Read the model definition and answer for the solid it produces. Units are mm, in the model's axes. Face numbers are marked on the shaded views. A direction names the side the tool comes from. Coordinates: 2 decimals unless noted, no trailing zeros. Loops run counter-clockwise (first coordinate to the right, second up) from the corner with the lowest first, then second, coordinate; pieces in that order, holes last. Notation, with made-up numbers: (-31, 45) -> (-26, 45) arc R7 cw to (-26, 51) -> close; hole circle Ø7 at (-13.75, -13). An arc over 180 degrees is marked (long way). Answer in a Markdown table with one row per item.
```python
from build123d import *

# Parameters (mm, degrees)
ESBO_O1_R                = 17.5
RESSALTO_EXTRUS_O1_DEPTH = 5
ESBO_O2_R                = 10
RESSALTO_EXTRUS_O2_DEPTH = 10
ESBO_O3_R                = 4
CORTE_EXTRUS_O1_DEPTH    = 16
ESBO_O4_R                = 1.5
CORTE_EXTRUS_O2_DEPTH    = 10
ESBO_O5_R                = 1.5
CORTE_EXTRUS_O3_DEPTH    = 18.5
ESBO_O6_R                = 1.5
CORTE_EXTRUS_O4_DEPTH    = 18.5


with BuildPart() as part:
    # Esboço1 → Ressalto-extrusão1 (new body)
    with BuildSketch(Plane(origin=(0, 0, 0), x_dir=(1, 0, 0), z_dir=(0, 1, 0))):
        Circle(ESBO_O1_R)
    extrude(amount=RESSALTO_EXTRUS_O1_DEPTH)

    # Esboço2 → Ressalto-extrusão2 (add)
    with BuildSketch(Plane(origin=(0, 5, 0), x_dir=(1, 0, 0), z_dir=(0, 1, 0))):
        Circle(ESBO_O2_R)
    extrude(amount=RESSALTO_EXTRUS_O2_DEPTH)

    # Esboço3 → Corte-extrusão1 (cut, through all)
    with BuildSketch(Plane(origin=(0, 15, 0), x_dir=(1, 0, 0), z_dir=(0, 1, 0))):
        Circle(ESBO_O3_R)
    extrude(amount=-CORTE_EXTRUS_O1_DEPTH, mode=Mode.SUBTRACT)

    # Esboço4 → Corte-extrusão2 (cut)
    with BuildSketch(Plane(origin=(0, 5, 0), x_dir=(1, 0, 0), z_dir=(0, 1, 0))):
        with Locations((0, 13.75)):
            Circle(ESBO_O4_R)
        with Locations((0, -13.75)):
            Circle(ESBO_O4_R)
    extrude(amount=-CORTE_EXTRUS_O2_DEPTH, mode=Mode.SUBTRACT)

    # Esboço5 → Corte-extrusão3 (cut, through all)
    with BuildSketch(Plane.XY):
        with Locations((0, 10)):
            Circle(ESBO_O5_R)
    extrude(amount=-CORTE_EXTRUS_O3_DEPTH, mode=Mode.SUBTRACT)

    # Esboço6 → Corte-extrusão4 (cut, through all)
    with BuildSketch(Plane(origin=(0, 0, 0), x_dir=(0, 0, -1), z_dir=(1, 0, 0))):
        with Locations((0, 10)):
            Circle(ESBO_O6_R)
    extrude(amount=-CORTE_EXTRUS_O4_DEPTH, mode=Mode.SUBTRACT)


solid = part.part
```
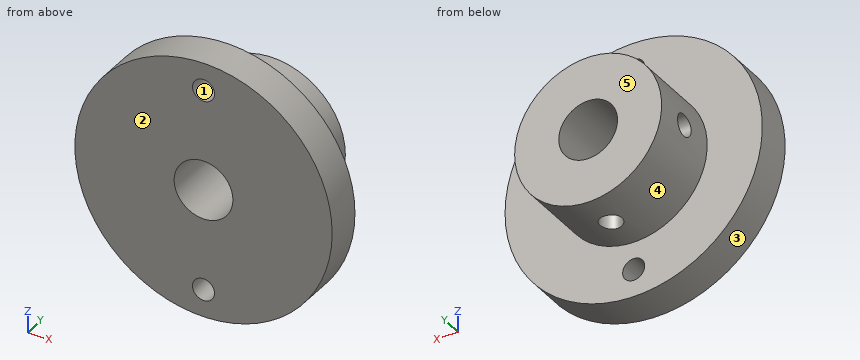
1. A tool of negligible diameter and unlimited length cuts with its end or side. For the marked faces 4 and 5, from which of +Z, -Z, +X, -X, +Y, -Y can it reach the whole face along a straight path? Write none if from no direction.
A:
| item | result |
|---|---|
| face 4 | +Y |
| face 5 | +Z, -Z, +X, -X, +Y |
2. A cutting plane is placed at B-B on x = 0. Give the vertices of the cut face in (y, z).
A:
| item | result |
|---|---|
| outline | (0, -17.5) -> (5, -17.5) -> (5, -15.25) -> (0, -15.25) -> close; (0, -12.25) -> (5, -12.25) -> (5, -10) -> (8.5, -10) -> (8.5, -4) -> (0, -4) -> close; (0, 4) -> (15, 4) -> (15, 10) -> (5, 10) -> (5, 12.25) -> (0, 12.25) -> close; (0, 15.25) -> (5, 15.25) -> (5, 17.5) -> (0, 17.5) -> close; (11.5, -10) -> (15, -10) -> (15, -4) -> (11.5, -4) -> close |
3. The mould has two halves that part along X. Classify the marked faces 1, 2 and 3: pulls with the +X half, pulls with the -X half, needs draft (parallel to the pull), parting line crosses it, or undercut.
A:
| item | result |
|---|---|
| face 1 | undercut |
| face 2 | needs draft |
| face 3 | parting line crosses it |
4. A cutting plane is placed at C-C on y = 10. Give the vertices of the cut face in (x, z).
A:
| item | result |
|---|---|
| outline | (-9.89, -1.5) arc R10 ccw to (-1.5, -9.89) -> (-1.5, -3.71) arc R4 cw to (-3.71, -1.5) -> close; (-9.89, 1.5) -> (-3.71, 1.5) arc R4 cw (long way) to (1.5, -3.71) -> (1.5, -9.89) arc R10 ccw (long way) to start |
5. Find the intervals of material crossed by probe 1 along Z at (x, y) = (0, 3.7); probe 2 along Y at (x, z) = (0, -8); probe 3 along Y at (x, z) = (-10, 13), in increasing order.
A:
| item | result |
|---|---|
| probe 1 | z = -17.5 to -15.25, -12.25 to -4, 4 to 12.25, 15.25 to 17.5 |
| probe 2 | y = 0 to 8.5, 11.5 to 15 |
| probe 3 | y = 0 to 5 |
6. A cutting plane is placed at D-D on z = 14.5. Give the vertices of the cut face in (x, y).
A:
| item | result |
|---|---|
| outline | (-9.8, 0) -> (-1.3, 0) -> (-1.3, 5) -> (-9.8, 5) -> close; (1.3, 0) -> (9.8, 0) -> (9.8, 5) -> (1.3, 5) -> close |
7. Given pin 1 Ø6 at (x, y) = (4.5, 6.5) entering from -Z; pin 2 Ø5 at (y, z) = (3.5, 6) entering from +X; pin 3 Ø1 at (x, y) = (0.5, 10.5) entering from -Z, each flat-ended and moving along its own axis, determine where each tip first touches the part or whether it passes through.
A:
| item | result |
|---|---|
| pin 1 | stops at z = -17.4 |
| pin 2 | stops at x = 17.15 |
| pin 3 | stops at z = 3.87 |
8. A cutting plane is placed at A-A on z = 0. Give the vertices of the cut face in (x, y).
A:
| item | result |
|---|---|
| outline | (-17.5, 0) -> (-4, 0) -> (-4, 8.5) -> (-10, 8.5) -> (-10, 5) -> (-17.5, 5) -> close; (-10, 11.5) -> (-4, 11.5) -> (-4, 15) -> (-10, 15) -> close; (4, 0) -> (17.5, 0) -> (17.5, 5) -> (10, 5) -> (10, 15) -> (4, 15) -> close |
